For this review, take the finished solid that the model builds, in its own axes (mm). Face numbers are marked on the shaded views. Give positions to 0.01 mm unless a question says otherwise; leave off trailing zeros. Order: outer loops, then holes, each group sorted by start corner. A loop starts at its lowest first (then second) coordinate and runs counter-clockwise, first axis right, second up. Notation, with made-up numbers: (-37, 45.5) -> (1, 45.5) arc R32 cw to (1, 81.5) -> close; hole circle Ø8 at (34.5, -12.5). An arc over 180 degrees is marked (long way). Use CSV: the item, a comma, the result in double quotes. Start each with the question number.
```python
from build123d import *

# Parameters (mm, degrees)
SKETCH1_R           = 16
SKETCH1_R_2         = 10
SKETCH1_R_3         = 2.5
BOSS_EXTRUDE1_DEPTH = 3
SCALE1_SCALE        = 1.9329
SCALE2_SCALE        = 1.5


with BuildPart() as part:
    # Sketch1 → Boss-Extrude1 (new body)
    with BuildSketch(Plane.XY):
        Circle(SKETCH1_R)
        Circle(SKETCH1_R_2, mode=Mode.SUBTRACT)
        with Locations((-13, 0)):
            Circle(SKETCH1_R_3, mode=Mode.SUBTRACT)
    extrude(amount=BOSS_EXTRUDE1_DEPTH)


with BuildPart() as part_1:
    # Scale1: scaled about (0.542570952, 0, 1.5)
    add(part.part.scale(SCALE1_SCALE).moved(Location((-0.506164441, 0, -1.39935))))


with BuildPart() as part_2:
    # Scale2: scaled about (0.542570951, 0, 1.5)
    add(part_1.part.scale(SCALE2_SCALE).moved(Location((-0.271285475, 0, -0.75))))


solid = part_2.part
```
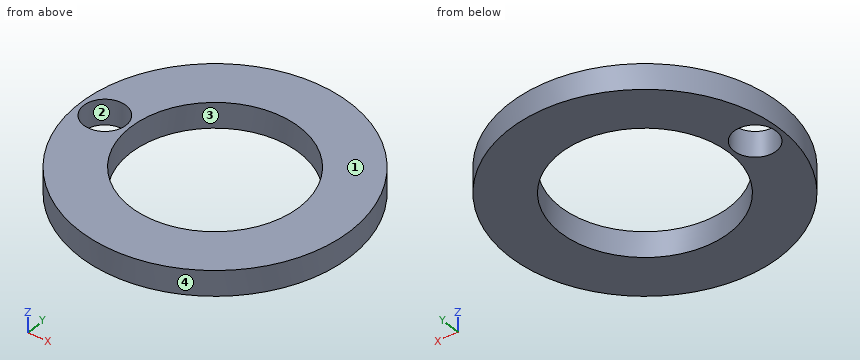
1. Draft analysis for pull direction X (two halves, no side actions). For the marked faces 1, 2, 3 and 4, state which applies: +X half, -X half, draft (parallel to the pull), parting line (faces both ways), or undercut.
2. Consider section D-D (z = 2.25). State the section outline as (x, y) points, plus the area to 3 significant figures.
3. Consider section A-A (y = 0). State the section outline as (x, z) points.
4. Clearance check with flat-ended pins moving along their axes: P1, Ø1, axis at x = 21, y = -15.5, coming from the -Z side; P2, Ø3, axis at x = -37.5, z = 2, coming from the -Y side; P3, Ø5, axis at y = 28, z = 0, coming from the +X side; P4, Ø4, axis at x = 1, z = 2, coming from the +Y side. State where each tip first meets the part, or that it passes through.
5. Consider section C-C (y = -18). State the section outline as (x, z) points.
6. To check wall thickness, follow L1, parallel to Y at x = -2, z = -1.75; L2, parallel to X at y = 2.5, z = -0.5; L3, parallel to Y at x = -3.5, z = 2.75. State the ranges of each line that lie inside material, in increasing order. Write a range as [from, to].
7. Consider section B-B (x = 15). State the section outline as (y, z) points, plus the area to 3 significant figures.
Answer list:
1,face 1,"draft"
1,face 2,"undercut"
1,face 3,"undercut"
1,face 4,"parting line"
2,outline,"circle Ø92.78 at (-1.03, 0); hole circle Ø14.5 at (-38.72, 0); hole circle Ø57.99 at (-1.03, 0)"
2,area,"3,950 mm2"
3,outline,"(-47.42, -2.85) -> (-45.97, -2.85) -> (-45.97, 5.85) -> (-47.42, 5.85) -> close; (-31.47, -2.85) -> (-30.02, -2.85) -> (-30.02, 5.85) -> (-31.47, 5.85) -> close; (27.96, -2.85) -> (45.36, -2.85) -> (45.36, 5.85) -> (27.96, 5.85) -> close"
4,P1,"through"
4,P2,"y = -30.48"
4,P3,"x = 37.72"
4,P4,"y = 46.39"
5,outline,"(-43.79, -2.85) -> (-23.76, -2.85) -> (-23.76, 5.85) -> (-43.79, 5.85) -> close; (21.7, -2.85) -> (41.72, -2.85) -> (41.72, 5.85) -> (21.7, 5.85) -> close"
6,L1,"[-46.38, -28.98], [28.98, 46.38]"
6,L2,"[-47.35, -45.53], [-31.92, -29.92], [27.85, 45.29]"
6,L3,"[-46.32, -28.89], [28.89, 46.32]"
7,outline,"(-43.53, -2.85) -> (-24.16, -2.85) -> (-24.16, 5.85) -> (-43.53, 5.85) -> close; (24.16, -2.85) -> (43.53, -2.85) -> (43.53, 5.85) -> (24.16, 5.85) -> close"
7,area,"337 mm2"
